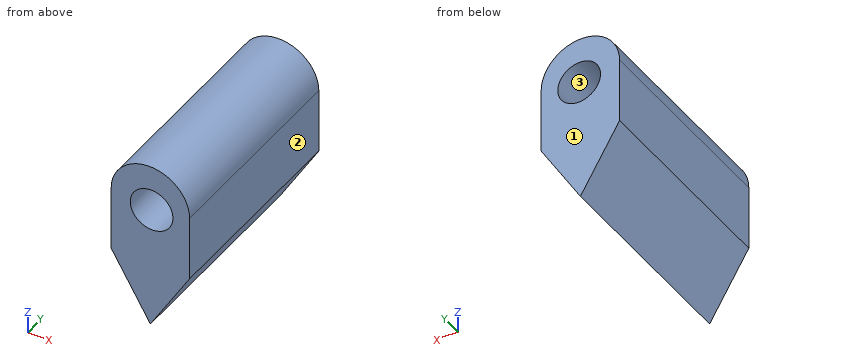
```python
from build123d import *

# Parameters (mm, degrees)
F1_DEPTH = 199.88325
F2_R     = 20.749815
F3_DEPTH = 239.77543


with BuildPart() as f1:
    # F0 (on Front) → F1 (new body)
    with BuildSketch(Plane.XZ):
        with BuildLine():
            Line((0, 63.5), (38.1, 0))
            Line((38.1, 0), (76.2, 63.5))
            Line((76.2, 63.5), (76.2, 127))
            ThreePointArc((76.2, 127), (38.1, 88.9), (0, 127))
            Line((0, 127), (0, 63.5))
        make_face()
        with BuildLine():
            Line((76.2, 127), (0, 127))
            ThreePointArc((0, 127), (38.1, 88.9), (76.2, 127))
        make_face()
        with BuildLine():
            ThreePointArc((76.2, 127), (38.1, 165.1), (0, 127))
            Line((0, 127), (76.2, 127))
        make_face()
    extrude(amount=F1_DEPTH)

    # F2 (on face) → F3 (cut)
    with BuildSketch(Plane(origin=(0, 0, 0), x_dir=(-1, 0, 0), z_dir=(0, 1, 0))):
        with Locations((-39.291214, 120.238699)):
            Circle(F2_R)
    extrude(amount=-F3_DEPTH, mode=Mode.SUBTRACT)


solid = f1.part
```
Build history of the part. All positions in model axes, mm. Face numbers are marked on the shaded views. Round coordinates to 2 decimals unless told otherwise and drop trailing zeros. Loops run counter-clockwise (first coordinate to the right, second up) from the corner with the lowest first, then second, coordinate; pieces in that order, holes last.
Item 1: Drill centre lines: line 1 along X through (y, z) = (-116, 139); line 2 along Z through (x, y) = (48.5, -186); line 3 along Z through (x, y) = (51.5, -42.5). Where is each one in solid material? Low to high.
Item 2: Saw through at A-A (x = 46). List the corners of the cut face in (y, z), then the cut area to 3 significant figures.
Item 3: Saw through at B-B (y = -185). List the corners of the cut face in (x, z), then the cut area to 3 significant figures.
Item 4: Two-plate mould, pull along X, no slides. Class the marked faces 1, 2 and 3: released by +X, released by -X, zero draft, split by the parting line, or undercut.
Item 5: Saw through at C-C (x = 33). List the corners of the cut face in (y, z).
Item 6: Saw through at D-D (x = 64). List the corners of the cut face in (y, z), then the cut area to 3 significant figures.
Item 7: Pin check, flat tips, straight feed: P1, Ø12, axis at y = -38.5, z = 141, coming from the +X side; P2, Ø1.5, axis at x = 17.5, y = -135.5, coming from the +Z side; P3, Ø3, axis at y = -84.5, z = 26, coming from the -X side. Stop position of each tip, or through.
Worked answers:
1. line 1: x = 1.94 to 30.43, 48.16 to 74.26
1. line 2: z = 17.33 to 101.64, 138.83 to 163.65
1. line 3: z = 22.33 to 103.46, 137.02 to 162.67
2. outline: (-199.88, 13.17) - (0, 13.17) - (0, 100.6) - (-199.88, 100.6) - close; (-199.88, 139.87) - (0, 139.87) - (0, 164.27) - (-199.88, 164.27) - close
2. area: 22,400 mm2
3. outline: (0, 63.5) - (38.1, 0) - (76.2, 63.5) - (76.2, 127) arc R38.1 ccw to (0, 127) - close; hole circle Ø41.5 at (39.29, 120.24)
3. area: 8,190 mm2
4. face 1: zero draft
4. face 2: released by +X
4. face 3: undercut
5. outline: (-199.88, 8.5) - (0, 8.5) - (0, 100.47) - (-199.88, 100.47) - close; (-199.88, 140.01) - (0, 140.01) - (0, 164.76) - (-199.88, 164.76) - close
6. outline: (-199.88, 43.17) - (0, 43.17) - (0, 154.94) - (-199.88, 154.94) - close
6. area: 22,300 mm2
7. P1: stops at x = 75.35
7. P2: stops at z = 159.52
7. P3: stops at x = 21.6
